For this review, use the dimensioned drawing (mm, ordinates from the lowest corner) and the shaded views. A direction names the side the tool comes from. Round coordinates to 2 decimals unless told otherwise and drop trailing zeros. Write each loop counter-clockwise with the first axis right and the second up, starting at its lowest first coordinate (ties: lowest second). Pieces come first, ordered by that corner, then holes. Notation, with made-up numbers: M 73.25,-30.75 L 121.25,-30.75 A9 ccw 121.25,-15.75 Z; hole C -8.5,82 d7. An arc over 180 degrees is marked long. Use one line per item in the form item = value. Start each with the question number.
Item 1: For line 1 (Z direction, x = 5, y = 14); line 2 (X direction, y = 22, z = 8.25); line 3 (Z direction, x = 12, y = 7.5), list the stretches that pass through material, from the lowest coordinate up. Write a range as [from, to].
Item 2: Add section D-D (x = 21.25). State the section outline as (y, z) points.
Item 3: Add section A-A (x = 6). State the section outline as (y, z) points.
Item 4: For P1, Ø5, axis at y = 19.5, z = 11, coming from the +X side; P2, Ø2, axis at x = 22, y = 21, coming from the +Z side; P3, Ø14, axis at x = 5, z = 14.5, coming from the -Y side; P4, Ø12, axis at y = 6.5, z = 14.5, coming from the -X side, all flat-tipped, find the tip position at first contact; note any pin that passes through.
Item 5: Add section B-B (y = 20.5). State the section outline as (x, z) points.
Item 6: For the marked faces 1, 2 and 3, list the 3-axis set-ups (+Z, -Z, +X, -X, +Y, -Y) from which the entire face can be reached by the end or side of a thin tool; tool diameter is ignored.
Item 7: Add section C-C (z = 17.75). State the section outline as (x, y) points.
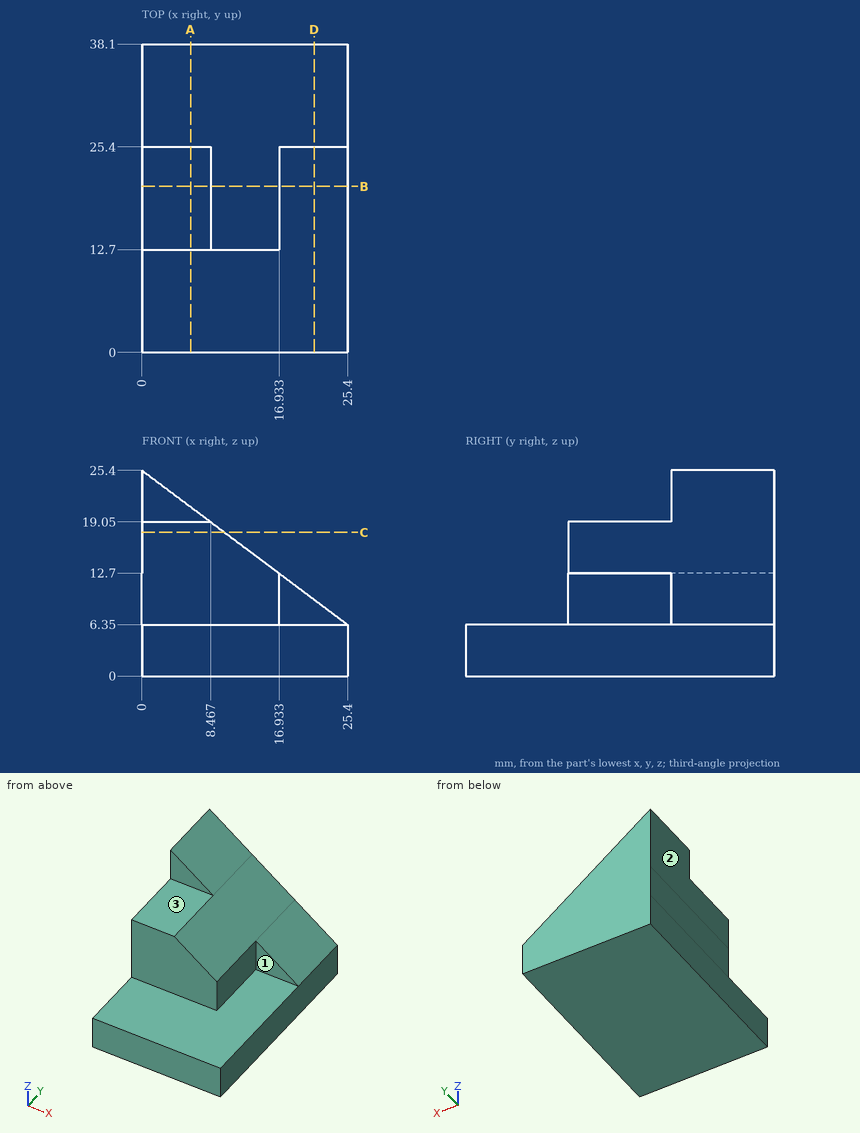
Calculated:
q1.line_1 = [0, 19.05]
q1.line_2 = [0, 16.93]
q1.line_3 = [0, 6.35]
q2.outline = M 0,0 L 38.1,0 L 38.1,9.46 L 25.4,9.46 L 25.4,6.35 L 0,6.35 Z
q3.outline = M 0,0 L 38.1,0 L 38.1,20.9 L 25.4,20.9 L 25.4,19.05 L 12.7,19.05 L 12.7,6.35 L 0,6.35 Z
q4.P1 = 16.93
q4.P2 = 6.35
q4.P3 = 12.7
q4.P4 = through
q5.outline = M 0,0 L 25.4,0 L 25.4,6.35 L 16.93,6.35 L 16.93,12.7 L 8.47,19.05 L 0,19.05 Z
q6.face_1 = +Z, +X, -Y
q6.face_2 = +Z, -Z, -X, +Y, -Y
q6.face_3 = +Z, +X, -X, -Y
q7.outline = M 0,12.7 L 10.2,12.7 L 10.2,38.1 L 0,38.1 Z
